Autodesk Inventor part; units mm, degrees
ref_plane "YZ Plane" through (0, 0, 0) normal (1, 0, 0) x (0, 1, 0)
ref_plane "XZ Plane" through (0, 0, 0) normal (0, 1, 0) x (-1, 0, 0)
ref_plane "XY Plane" through (0, 0, 0) normal (0, 0, 1) x (1, 0, 0)
sketch "スケッチ1" plane through (0, 0, 0) normal (0, 1, 0) x (-1, 0, 0)
  line L0 (-5.08, 7.62) -> (5.08, 7.62)
  line L1 (5.08, 7.62) -> (5.08, -7.62)
  line L2 (5.08, -7.62) -> (-5.08, -7.62)
  line L3 (-5.08, -7.62) -> (-5.08, 7.62)
  line L4 (-5.08, 7.62) -> (5.08, -7.62) construction
  line L5 (5.08, 7.62) -> (-5.08, -7.62) construction
  point P0 (0, 0)
  dimension "d0" = 10.16
  dimension "d1" = 15.24
extrude "押し出し1" add sketch "スケッチ1" along normal blind 1.6
sketch "スケッチ2" plane through (0, 1.6, 0) normal (0, 1, 0) x (1, 0, 0)
  line L0 (2, -2.75) -> (-2, -2.75)
  line L1 (-2, -2.75) -> (-2, 2.75)
  line L2 (-2, 2.75) -> (2, 2.75)
  line L3 (2, 2.75) -> (2, -2.75)
  line L4 (2, -2.75) -> (-2, 2.75) construction
  line L5 (-2, -2.75) -> (2, 2.75) construction
  point P0 (0, 0)
  dimension "d4" = 4
  dimension "d5" = 5.5
extrude "押し出し2" add sketch "スケッチ2" along normal blind 1
sketch "スケッチ3" plane through (0, 0, 0) normal (0, -1, 0) x (1, 0, 0)
  line L0 (2.54, 6.35) -> (5.08, 6.35)
  line L1 (5.08, 6.35) -> (5.08, 3.81)
  line L2 (5.08, 3.81) -> (2.54, 3.81)
  line L3 (2.54, 3.81) -> (2.54, 6.35)
  line L4 (2.54, 6.35) -> (5.08, 3.81) construction
  line L5 (5.08, 6.35) -> (2.54, 3.81) construction
  line L6 (1.5528, 5.08) -> (3.81, 2.8228)
  line L7 (3.81, 2.8228) -> (6.0672, 5.08)
  line L8 (6.0672, 5.08) -> (3.81, 7.3372)
  line L9 (3.81, 7.3372) -> (1.5528, 5.08)
  line L10 (1.5528, 5.08) -> (6.0672, 5.08) construction
  line L11 (3.81, 2.8228) -> (3.81, 7.3372) construction
  point P0 (0, 0)
  point P1 (3.81, 5.08)
  point P2 (3.81, 5.08)
  point P3 (3.81, 5.08)
  point P4 (2.8228, 6.35)
  point P5 (2.54, 6.0672)
  point P6 (2.54, 4.0928)
  point P7 (2.8228, 3.81)
  point P8 (4.7972, 3.81)
  point P9 (5.08, 4.0928)
  point P10 (5.08, 6.0672)
  point P11 (4.7972, 6.35)
  dimension "d8" = 2.54
  dimension "d9" = 2.54
  dimension "d10" = 5.08
  dimension "d11" = 3.81
  dimension "d31" = 0.2
extrude "押し出し3" add sketch "スケッチ3" along normal blind 2.5 contours L0 L8 L1 L7 L2 L6 L3 L9
sketch "スケッチ4" plane through (0, -2.5, 0) normal (0, -1, 0) x (1, 0, 0)
  line L0 (4.7972, 6.35) -> (2.8228, 6.35)
  line L1 (5.08, 4.0928) -> (5.08, 6.0672)
  circle A0 centre (3.81, 5.08) radius 0.5
  point P0 (0, 0)
  point P1 (4.88, 6.35)
  point P2 (2.74, 6.35)
  point P3 (5.08, 4.01)
  point P4 (5.08, 6.15)
  point P5 (5.08, 5.08)
  point P6 (3.81, 6.35)
  point P7 (5.08, 6.35)
  point P8 (2.54, 6.35)
  point P9 (5.08, 3.81)
  dimension "d17" = 1
extrude "押し出し4" add sketch "スケッチ4" along normal blind 7
sketch "スケッチ5" plane through (0, 1.6, 0) normal (0, 1, 0) x (1, 0, 0)
  circle A0 centre (3.81, -5.08) radius 0.5
  circle A1 centre (3.81, -5.08) radius 0.5
  point P0 (0, 0)
extrude "押し出し5" add sketch "スケッチ5" along normal blind 1
pattern_linear "矩形状パターン2" count 5 spacing 2.54 along (0, 0, -1) count 2 spacing 7.62 along (-1, 0, 0) of "押し出し3", "押し出し4", "押し出し5"
properties part number "bno055_module"
The model under review builds one solid part; all positions refer to its coordinate system, in mm. A direction names the side the tool comes from. Round coordinates to 2 decimals unless told otherwise and drop trailing zeros. Order: outer loops, then holes, each group sorted by start corner. A loop starts at its lowest first (then second) coordinate and runs counter-clockwise, first axis right, second up. Notation, with made-up numbers: (8, 75) -> (46, 75) arc R23 ccw to (46, 102) -> close; hole circle Ø4 at (34.25, 57). An arc over 180 degrees is marked (long way). Use a Markdown table: item, result.
Q1. For line 1 (Z direction, x = -3.75, y = -7.75); line 2 (X direction, y = -2.25, z = 4.75); line 3 (Z direction, x = -3.75, y = -1), list the stretches that pass through material, from the lowest coordinate up.
Values:
| item | result |
|---|---|
| line 1 | z = -5.58 to -4.58, -3.04 to -2.04, -0.5 to 0.5, 2.04 to 3.04, 4.58 to 5.58 |
| line 2 | x = -5.08 to -2.54, 2.54 to 5.08 |
| line 3 | z = -6.35 to 6.35 |
Q2. Tool access review of faces 5 (the cylindrical face through (3.41, -5.95, -4.78)), 6 (the cylindrical face through (-3.918, 2.093, 4.592)), 7 (the flat face through (2.54, -1, -3)): name each direction out of +Z, -Z, +X, -X, +Y, -Y from which nothing blocks a thin tool from reaching the whole face with its end or side.
Values:
| item | result |
|---|---|
| face 5 | -Y |
| face 6 | +Y |
| face 7 | +Z, -Z, -Y |
Q3. Clearance check with flat-ended pins moving along their axes: P1, Ø0.6, axis at x = -3.5, y = -1.5, coming from the +Z side; P2, Ø2, axis at x = -4, y = -2, coming from the -Z side; P3, Ø2, axis at x = -4.5, z = -3, coming from the -Y side; P4, Ø3, axis at x = -2, z = -1.5, coming from the -Y side. State where each tip first meets the part, or that it passes through.
Values:
| item | result |
|---|---|
| P1 | stops at z = 6.35 |
| P2 | stops at z = -6.35 |
| P3 | stops at y = -9.5 |
| P4 | stops at y = -2.5 |
Q4. We need section C-C on x = 4.5. Write out the cut boundary in (y, z), then the cut area to 3 significant figures.
Values:
| item | result |
|---|---|
| outline | (-2.5, -6.35) -> (0, -6.35) -> (0, -7.62) -> (1.6, -7.62) -> (1.6, 7.62) -> (0, 7.62) -> (0, 6.35) -> (-2.5, 6.35) -> close |
| area | 56.1 mm^2 |
Q5. We need section A-A on y = -5.5. State how many separate pieces and enclosed holes the cut face has, then the cut area to 3 significant figures.
Values:
| item | result |
|---|---|
| separate pieces | 10 |
| enclosed holes | 0 |
| area | 7.85 mm^2 |
Q6. We need section B-B on z = -5.08. Write out the cut boundary in (x, y), then the cut area to 3 significant figures.
Values:
| item | result |
|---|---|
| outline | (-5.08, -2.5) -> (-4.31, -2.5) -> (-4.31, -9.5) -> (-3.31, -9.5) -> (-3.31, -2.5) -> (-2.54, -2.5) -> (-2.54, 0) -> (2.54, 0) -> (2.54, -2.5) -> (3.31, -2.5) -> (3.31, -9.5) -> (4.31, -9.5) -> (4.31, -2.5) -> (5.08, -2.5) -> (5.08, 1.6) -> (4.31, 1.6) -> (4.31, 2.6) -> (3.31, 2.6) -> (3.31, 1.6) -> (-3.31, 1.6) -> (-3.31, 2.6) -> (-4.31, 2.6) -> (-4.31, 1.6) -> (-5.08, 1.6) -> close |
| area | 45.0 mm^2 |
Q7. Mouldability with a two-part tool opening along Z and no side actions: class faces 1 (the cylindrical face through (-4.179, -5.951, 2.202)), 2 (the cylindrical face through (3.441, -5.951, 2.202)), 3 (the flat face through (0, 1, 7.62)), 4 (the flat face through (4, -9.5, -5)) as +Z half, -Z half, draft (parallel to the pull), parting line (faces both ways), or undercut.
Values:
| item | result |
|---|---|
| face 1 | undercut |
| face 2 | undercut |
| face 3 | +Z half |
| face 4 | draft |
Q8. We need section D-D on z = -2.54. Write out the cut boundary in (x, y).
Values:
| item | result |
|---|---|
| outline | (-5.08, -2.5) -> (-4.31, -2.5) -> (-4.31, -9.5) -> (-3.31, -9.5) -> (-3.31, -2.5) -> (-2.54, -2.5) -> (-2.54, 0) -> (2.54, 0) -> (2.54, -2.5) -> (3.31, -2.5) -> (3.31, -9.5) -> (4.31, -9.5) -> (4.31, -2.5) -> (5.08, -2.5) -> (5.08, 1.6) -> (4.31, 1.6) -> (4.31, 2.6) -> (3.31, 2.6) -> (3.31, 1.6) -> (2, 1.6) -> (2, 2.6) -> (-2, 2.6) -> (-2, 1.6) -> (-3.31, 1.6) -> (-3.31, 2.6) -> (-4.31, 2.6) -> (-4.31, 1.6) -> (-5.08, 1.6) -> close |
